from build123d import *

# Parameters (mm, degrees)
F0_W     = 2.5
F0_H     = 58.5
F1_DEPTH = 32.5
F3_DEPTH = 5
F4_R     = 2.5
F5_DEPTH = 5


with BuildPart() as f1:
    # F0 (on Right) → F1 (new body, symmetric)
    with BuildSketch(Plane.YZ):
        Polygon((0, 2.5), (0, 0), (2.5, 0), (37, 0), (37, 2.5), align=None)
        with Locations((1.25, -29.25)):
            Rectangle(F0_W, F0_H)
    extrude(amount=F1_DEPTH, both=True)

    # F2 (on Front) → F3 (cut, symmetric)
    with BuildSketch(Plane.XZ):
        with BuildLine():
            Line((-26.5, -31.5), (-26.5, -26.5))
            ThreePointArc((-26.5, -26.5), (-29, -29), (-26.5, -31.5))
        make_face()
        with BuildLine():
            ThreePointArc((-26.5, -31.5), (-24.732233047, -30.767766953), (-24, -29))
            ThreePointArc((-24, -29), (-24.732233047, -27.232233047), (-26.5, -26.5))
            Line((-26.5, -26.5), (-26.5, -31.5))
        make_face()
        with BuildLine():
            Line((-8.5, -31.5), (-8.5, -26.5))
            ThreePointArc((-8.5, -26.5), (-11, -29), (-8.5, -31.5))
        make_face()
        with BuildLine():
            ThreePointArc((-8.5, -31.5), (-6.732233047, -30.767766953), (-6, -29))
            ThreePointArc((-6, -29), (-6.732233047, -27.232233047), (-8.5, -26.5))
            Line((-8.5, -26.5), (-8.5, -31.5))
        make_face()
        with BuildLine():
            Line((8.5, -31.5), (8.5, -26.5))
            ThreePointArc((8.5, -26.5), (6, -29), (8.5, -31.5))
        make_face()
        with BuildLine():
            ThreePointArc((8.5, -31.5), (10.267766953, -30.767766953), (11, -29))
            ThreePointArc((11, -29), (10.267766953, -27.232233047), (8.5, -26.5))
            Line((8.5, -26.5), (8.5, -31.5))
        make_face()
        with BuildLine():
            Line((26.5, -31.5), (26.5, -26.5))
            ThreePointArc((26.5, -26.5), (24, -29), (26.5, -31.5))
        make_face()
        with BuildLine():
            ThreePointArc((26.5, -31.5), (28.267766953, -30.767766953), (29, -29))
            ThreePointArc((29, -29), (28.267766953, -27.232233047), (26.5, -26.5))
            Line((26.5, -26.5), (26.5, -31.5))
        make_face()
        with BuildLine():
            Line((-26.5, -55.5), (-26.5, -50.5))
            ThreePointArc((-26.5, -50.5), (-29, -53), (-26.5, -55.5))
        make_face()
        with BuildLine():
            ThreePointArc((-24, -53), (-24.732233047, -51.232233047), (-26.5, -50.5))
            Line((-26.5, -50.5), (-26.5, -55.5))
            ThreePointArc((-26.5, -55.5), (-24.732233047, -54.767766953), (-24, -53))
        make_face()
        with BuildLine():
            ThreePointArc((-6, -53), (-6.732233047, -51.232233047), (-8.5, -50.5))
            Line((-8.5, -50.5), (-8.5, -55.5))
            ThreePointArc((-8.5, -55.5), (-6.732233047, -54.767766953), (-6, -53))
        make_face()
        with BuildLine():
            Line((-8.5, -55.5), (-8.5, -50.5))
            ThreePointArc((-8.5, -50.5), (-11, -53), (-8.5, -55.5))
        make_face()
        with BuildLine():
            ThreePointArc((11, -53), (10.267766953, -51.232233047), (8.5, -50.5))
            Line((8.5, -50.5), (8.5, -55.5))
            ThreePointArc((8.5, -55.5), (10.267766953, -54.767766953), (11, -53))
        make_face()
        with BuildLine():
            Line((8.5, -55.5), (8.5, -50.5))
            ThreePointArc((8.5, -50.5), (6, -53), (8.5, -55.5))
        make_face()
        with BuildLine():
            ThreePointArc((29, -53), (28.267766953, -51.232233047), (26.5, -50.5))
            Line((26.5, -50.5), (26.5, -55.5))
            ThreePointArc((26.5, -55.5), (28.267766953, -54.767766953), (29, -53))
        make_face()
        with BuildLine():
            Line((26.5, -55.5), (26.5, -50.5))
            ThreePointArc((26.5, -50.5), (24, -53), (26.5, -55.5))
        make_face()
    extrude(amount=F3_DEPTH, both=True, mode=Mode.SUBTRACT)

    # F4 (on face) → F5 (cut, symmetric)
    with BuildSketch(Plane.XY.offset(2.5)):
        with Locations((-26.5, 7.894)):
            Circle(F4_R)
        with Locations((-26.5, 31.894)):
            Circle(F4_R)
        with Locations((-8.5, 31.894)):
            Circle(F4_R)
        with Locations((-8.5, 7.894)):
            Circle(F4_R)
        with Locations((8.5, 7.894)):
            Circle(F4_R)
        with Locations((8.5, 31.8015553057)):
            Circle(F4_R)
        with Locations((26.5, 31.894)):
            Circle(F4_R)
        with Locations((26.5, 7.894)):
            Circle(F4_R)
    extrude(amount=F5_DEPTH, both=True, mode=Mode.SUBTRACT)


solid = f1.part
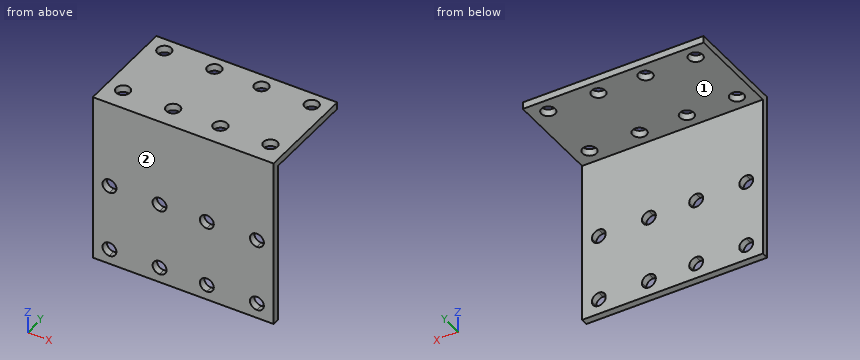
Geometry check sheet. Reference: the model listing, model coordinates, mm. Face numbers are marked on the shaded views. A direction names the side the tool comes from. Give positions to 0.01 mm unless a question says otherwise; leave off trailing zeros. Loops run counter-clockwise (first coordinate to the right, second up) from the corner with the lowest first, then second, coordinate; pieces in that order, holes last.
(1) Section check C-C on y = 3.5. Record the cut outline in (x, z), then the cut area to 4 significant figures.
From the geometry:
outline: (-32.5, 0) - (32.5, 0) - (32.5, 2.5) - (-32.5, 2.5) - close
area: 162.5 mm2
(2) Section check B-B on x = -10. Record the cut outline in (y, z), then the cut area to 3 significant figures.
From the geometry:
outline: (0, -58.5) - (2.5, -58.5) - (2.5, -55) - (0, -55) - close; (0, -51) - (2.5, -51) - (2.5, -31) - (0, -31) - close; (0, -27) - (2.5, -27) - (2.5, 0) - (5.89, 0) - (5.89, 2.5) - (0, 2.5) - close; (9.89, 0) - (29.89, 0) - (29.89, 2.5) - (9.89, 2.5) - close; (33.89, 0) - (37, 0) - (37, 2.5) - (33.89, 2.5) - close
area: 199 mm2
(3) Set-up check for the marked faces 1 and 2: record each of +Z, -Z, +X, -X, +Y, -Y from which the full face is reachable in a straight line by a thin tool's end or side.
From the geometry:
face 1: -Z, +X, -X, +Y
face 2: +Z, -Z, +X, -X, -Y
(4) Depth check by flat-ended pin: pin 1 Ø1.5 at (x, z) = (17.5, -9) entering from +Y; pin 2 Ø5 at (x, z) = (25, -10) entering from -Y; pin 3 Ø6 at (x, y) = (-6.5, 14) entering from -Z. Enter the tip coordinate at first touch or a pass-through.
From the geometry:
pin 1: stops at y = 2.5
pin 2: stops at y = 0
pin 3: stops at z = 0
(5) Thickness scan on L1, parallel to Y at x = -26.5, z = 1.8; L2, parallel to Y at x = 8, z = 1; L3, parallel to Z at x = 24, y = 22.5. Record the ranges inside material, lowest first.
From the geometry:
L1: y = 0 to 5.39, 10.39 to 29.39, 34.39 to 37
L2: y = 0 to 5.44, 10.34 to 29.35, 34.25 to 37
L3: z = 0 to 2.5
(6) Section check A-A on x = 1.5. Record the cut outline in (y, z), then the cut area to 3 significant figures.
From the geometry:
outline: (0, -58.5) - (2.5, -58.5) - (2.5, 0) - (37, 0) - (37, 2.5) - (0, 2.5) - close
area: 239 mm2
